```python
from build123d import *

# Parameters (mm, degrees)
F1_DEPTH  = 60
F3_DEPTH  = 10
F4_DEPTH  = 30
F6_DEPTH  = 50
F8_DEPTH  = 25
F9_R      = 5
F10_DEPTH = 25
F11_R     = 10


with BuildPart() as f1:
    # F0 (on Front) → F1 (new body)
    with BuildSketch(Plane.XZ):
        with BuildLine():
            Line((-34.3805874884, -42.3699883783), (-54.3805874884, -42.3699883783))
            Line((-54.3805874884, -42.3699883783), (-54.3805874884, -52.3699883783))
            Line((-54.3805874884, -52.3699883783), (-24.3805874884, -52.3699883783))
            Line((-24.3805874884, -52.3699883783), (-24.3805874884, -42.3699883783))
            ThreePointArc((-24.3805874884, -42.3699883783), (5.6194125116, -12.3699883783), (35.6194125116, -42.3699883783))
            Line((35.6194125116, -42.3699883783), (35.6194125116, -52.3699883783))
            Line((35.6194125116, -52.3699883783), (65.6194125116, -52.3699883783))
            Line((65.6194125116, -52.3699883783), (65.6194125116, -42.3699883783))
            Line((65.6194125116, -42.3699883783), (45.6194125116, -42.3699883783))
            ThreePointArc((45.6194125116, -42.3699883783), (5.6194125116, -2.3699883783), (-34.3805874884, -42.3699883783))
        make_face()
    extrude(amount=F1_DEPTH)

    # F2 (on face) → F3 (join)
    with BuildSketch(Plane(origin=(0, 0, 0), x_dir=(-1, 0, 0), z_dir=(0, 1, 0))):
        with BuildLine():
            ThreePointArc((19.3804243856, 57.7203172984), (-5.6194125116, 32.6300116217), (-30.6192494088, 57.7203172984))
            Line((-30.6192494088, 57.7203172984), (-43.8620893558, -30.6440484251))
            ThreePointArc((-43.8620893558, -30.6440484251), (-5.6194125116, -2.3699883783), (32.6232643327, -30.6440484251))
            Line((32.6232643327, -30.6440484251), (19.3804243856, 57.7203172984))
        make_face()
    extrude(amount=-F3_DEPTH)

    # F2 (on face) → F4 (join)
    with BuildSketch(Plane(origin=(0, 0, 0), x_dir=(-1, 0, 0), z_dir=(0, 1, 0))):
        with BuildLine():
            ThreePointArc((9.3803156488, 57.7203172984), (-5.6194125116, 42.6300116217), (-20.6191406719, 57.7203172984))
            Line((-20.6191406719, 57.7203172984), (-30.6192494088, 57.7203172984))
            ThreePointArc((-30.6192494088, 57.7203172984), (-5.6194125116, 32.6300116217), (19.3804243856, 57.7203172984))
            Line((19.3804243856, 57.7203172984), (9.3803156488, 57.7203172984))
        make_face()
    extrude(amount=-F4_DEPTH)

    # F5 (on face) → F6 (join, through all)
    with BuildSketch(Plane.XZ.offset(10)):
        with BuildLine():
            ThreePointArc((10.6194125116, 33.1351141939), (5.6194125116, 32.6300116217), (0.6194125116, 33.1351141939))
            Line((0.6194125116, 33.1351141939), (0.6194125116, -2.6837187123))
            ThreePointArc((0.6194125116, -2.6837187123), (5.6194125116, -2.3699883783), (10.6194125116, -2.6837187123))
            Line((10.6194125116, -2.6837187123), (10.6194125116, 33.1351141939))
        make_face()
    extrude(amount=F6_DEPTH)

    # F7 (on face) → F8 (cut)
    with BuildSketch(Plane.YZ.offset(10.6194125116)):
        Polygon((-60, -2.6837187123), (-30, 33.1351141939), (-60, 33.1351141939), align=None)
    extrude(amount=-F8_DEPTH, mode=Mode.SUBTRACT)

    # F9 (on face) → F10 (cut)
    with BuildSketch(Plane.XY.offset(-42.3699883783)):
        with Locations((55.6194125116, -50)):
            Circle(F9_R)
        with Locations((55.6194125116, -10)):
            Circle(F9_R)
        with Locations((-44.3805874884, -50)):
            Circle(F9_R)
        with Locations((-44.3805874884, -10)):
            Circle(F9_R)
    extrude(amount=-F10_DEPTH, mode=Mode.SUBTRACT)

    # F11
    f11_edges = [f1.edges().sort_by_distance(p)[0] for p in [
        (65.619413, -60, -47.369988),
        (65.619413, 0, -47.369988),
        (-54.380587, -60, -47.369988),
        (-54.380587, 0, -47.369988),
    ]]
    fillet(f11_edges, radius=F11_R)


solid = f1.part
```
Input: part model. Units: mm. Frame: model coordinates. A direction names the side the tool comes from. Give positions to 0.01 mm unless a question says otherwise; leave off trailing zeros. Loops run counter-clockwise (first coordinate to the right, second up) from the corner with the lowest first, then second, coordinate; pieces in that order, holes last. Notation, with made-up numbers: M 71,55.5 L 112,55.5 A14 ccw 112,77.5 Z; hole C 56,-3.5 d3. An arc over 180 degrees is marked long. Answer as CSV lines item,"result". Start each with the question number.
1. Section D-D on z = 19.5. Return loops of the section in (x, y).
2. Pin query (flat end, axial travel): P1, Ø6, axis at x = 27.5, y = -34, coming from the +Z side; P2, Ø18, axis at y = -36.5, z = 23, coming from the +X side; P3, Ø11.5, axis at x = -44.38, y = -10, coming from the -Z side; P4, Ø5, axis at x = 3.5, z = 35.5, coming from the -Y side. Return the tip coordinate at first contact, or that it passes through.
3. Reachability of faces 4 (the face through (-24.381, -30, -47)), 5 (the face through (56, -30, -42.37)), 6 (the face through (-44, -30, -42.37)), 7 (the face through (-24.1, -36.2, -15.6)) from +Z, -Z, +X, -X, +Y, -Y: full face, straight path, thin tool, end or side. Return the list, or none.
4. Line query: L1, parallel to Y at x = 24, z = 10.5; L2, parallel to Z at x = -42.5, y = -23.5; L3, parallel to Z at x = 23.5, y = -13. Output: solid intervals per line, ascending.
5. Pull-direction query (X, two-part tool) for faces 1 (the face through (51.934, -46.621, -47.3)), 2 (the face through (6, 0, 3)), 3 (the face through (37.148, -4.93, 14.157)); classes: released by +X, released by -X, zero draft, split by the parting line, or undercut.
6. Section C-C on y = -41. Return loops of the section in (x, z), plus the area to 3 significant figures.
7. Section B-B on x = 40. Return loops of the section in (y, z), plus the area to 3 significant figures.
8. Section A-A on z = -24. Return loops of the section in (x, y).
Computed values:
1,outline,"M -25.11,-10 L 0.62,-10 L 0.62,-41.42 L 10.62,-41.42 L 10.62,-10 L 36.35,-10 L 36.35,0 L -25.11,0 Z"
2,P1,"stops at z = -7.11"
2,P2,"stops at x = 10.62"
2,P3,"stops at z = -52.37"
2,P4,"stops at y = -30"
3,face 4,"-Z, +Y, -Y"
3,face 5,"+Z, +X, +Y, -Y"
3,face 6,"+Z, -X, +Y, -Y"
3,face 7,"-X, -Y"
4,L1,"y = -10 to 0"
4,L2,"z = -52.37 to -42.37"
4,L3,"z = -18.28 to -6.59, 40.16 to 57.72"
5,face 1,"undercut"
5,face 2,"zero draft"
5,face 3,"released by +X"
6,outline,"M -54.38,-52.37 L -24.38,-52.37 L -24.38,-42.37 A30 cw 35.62,-42.37 L 35.62,-52.37 L 65.62,-52.37 L 65.62,-42.37 L 45.62,-42.37 A40 ccw 10.62,-2.68 L 10.62,20 L 0.62,20 L 0.62,-2.68 A40 ccw -34.38,-42.37 L -54.38,-42.37 Z"
6,area,"1,920 mm²"
7,outline,"M -60,-52.37 L 0,-52.37 L 0,-4.87 L -10,-4.87 L -10,-21.93 L -60,-21.93 Z"
7,area,"2,000 mm²"
8,outline,"M -31.63,-10 L -29.91,-10 L -29.91,-60 L -18.1,-60 L -18.1,0 L -31.63,0 Z; M 29.34,-60 L 41.15,-60 L 41.15,-10 L 42.87,-10 L 42.87,0 L 29.34,0 Z"
